For this review, take the finished solid that the model builds, in its own axes (mm). A direction names the side the tool comes from. Give positions to 0.01 mm unless a question says otherwise; leave off trailing zeros. Write each loop counter-clockwise with the first axis right and the second up, starting at its lowest first coordinate (ties: lowest second). Pieces come first, ordered by that corner, then holes. Notation, with made-up numbers: M 24.5,79.25 L 70.5,79.25 A15 ccw 70.5,93.25 Z; hole C 57.5,56.5 d11. An arc over 180 degrees is marked long. Write item = value, one per line.
```python
from build123d import *

# Parameters (mm, degrees)
BOSS_EXTRUDE1_DEPTH = 10


with BuildPart() as part:
    # Sketch1 → Boss-Extrude1 (new, symmetric)
    with BuildSketch(Plane(origin=(0, 0, 0), x_dir=(1, 0, 0), z_dir=(0, 1, 0))):
        with BuildLine():
            Line((1.29375, 0), (1.29375, -4.5))
            Line((1.29375, -4.5), (0.5, -4.5))
            Line((0.5, -4.5), (0.5, 0))
            ThreePointArc((0.5, 0), (0.353553391, 0.353553391), (0, 0.5))
            Line((0, 0.5), (-1.20625, 0.5))
            ThreePointArc((-1.20625, 0.5), (-2.441545823, 1.409259047), (-1.940487786, 2.858965441))
            Line((-1.940487786, 2.858965441), (1.559512214, 5.271465441))
            ThreePointArc((1.559512214, 5.271465441), (2.714013578, 5.429837997), (3.52755254, 4.595506155))
            Line((3.52755254, 4.595506155), (4.524019527, 1.437062839))
            ThreePointArc((4.524019527, 1.437062839), (5.076956782, 1.093325967), (5.500851427, 1.5875))
            Line((5.500851427, 1.5875), (5.500851427, 5.5))
            Line((5.500851427, 5.5), (6.294601427, 5.5))
            Line((6.294601427, 5.5), (6.294601427, 1.5875))
            ThreePointArc((6.294601427, 1.5875), (5.197774033, 0.30882469), (3.767048886, 1.198243845))
            Line((3.767048886, 1.198243845), (2.7705819, 4.356687161))
            ThreePointArc((2.7705819, 4.356687161), (2.456170707, 4.67913425), (2.009986604, 4.617927465))
            Line((2.009986604, 4.617927465), (-1.490013396, 2.205427465))
            ThreePointArc((-1.490013396, 2.205427465), (-1.683659014, 1.645154463), (-1.20625, 1.29375))
            Line((-1.20625, 1.29375), (0, 1.29375))
            ThreePointArc((0, 1.29375), (0.914819398, 0.914819398), (1.29375, 0))
        make_face()
    extrude(amount=BOSS_EXTRUDE1_DEPTH, both=True)


solid = part.part
```
1. For line 1 along X through (y, z) = (-4.75, -3.5); line 2 along X through (y, z) = (4.5, -2.5); line 3 along X through (y, z) = (7, 3.5), list the stretches that pass through material, from the lowest coordinate up. Write a range as from..to.
Responses:
line_1 = -1.01..0.39, 3.04..3.87, 5.5..6.29
line_2 = -2.29..-1.06, 3.36..4.19, 5.5..6.29
line_3 = 0.5..1.29
2. Insertion check: P1, Ø5, axis at y = 0, z = 2, coming from the +X side; P2, Ø2, axis at y = 4.5, z = 1, coming from the -X side; P3, Ø3, axis at y = 6.5, z = 3.5, coming from the +X side. Each pin has a flat end and moves straight along its axis. Give the tip position at first contact, or say it passes through.
Responses:
P1 = 5.7
P2 = 0.5
P3 = 1.29
3. Machinability: for faces 1 (the face through (3.276, 0.14, -2.755)), 2 (the face through (4.02, 0.14, -3.04)), 3 (the face through (0.5, 0, 2)), 4 (the face through (0.284, 0.14, -3.429)), which of the approach directions +Z, -Z, +X, -X, +Y, -Y give a long, thin tool a straight path to every point of the face, cutting with its end or side? Answer none if there is none.
Responses:
face_1 = +Z, +Y, -Y
face_2 = -Z, +Y, -Y
face_3 = +Z, -X, +Y, -Y
face_4 = +Y, -Y
4. The part is to be moulded in two halves that separate along Z. For faces 5 (the face through (0.905, 0.14, -0.925)), 6 (the face through (5.501, 0, -4)), 7 (the face through (2.698, 0.14, -5.435)), say which applies: +Z half, -Z half, draft (parallel to the pull), parting line (faces both ways), or undercut.
Responses:
face_5 = undercut
face_6 = draft
face_7 = -Z half
5. We need section B-B, the plane x = -0.5. Write out the cut boundary in (y, z).
Responses:
outline = M -10,-3.85 L 10,-3.85 L 10,-2.89 L -10,-2.89 Z; M -10,-1.29 L 10,-1.29 L 10,-0.5 L -10,-0.5 Z
6. We need section D-D, the plane z = 3. Write out the cut boundary in (x, y).
Responses:
outline = M 0.5,-10 L 1.29,-10 L 1.29,10 L 0.5,10 Z
7. We need section C-C, the plane z = -3.25. Write out the cut boundary in (x, y).
Responses:
outline = M -1.37,-10 L 0.03,-10 L 0.03,10 L -1.37,10 Z; M 3.12,-10 L 3.95,-10 L 3.95,10 L 3.12,10 Z; M 5.5,-10 L 6.29,-10 L 6.29,10 L 5.5,10 Z
8. We need section A-A, the plane y = -1.5. Write out the cut boundary in (x, z).
Responses:
outline = M -1.94,-2.86 L 1.56,-5.27 A1.29 ccw 3.53,-4.6 L 4.52,-1.44 A0.5 cw 5.5,-1.59 L 5.5,-5.5 L 6.29,-5.5 L 6.29,-1.59 A1.29 ccw 3.77,-1.2 L 2.77,-4.36 A0.5 cw 2.01,-4.62 L -1.49,-2.21 A0.5 cw -1.21,-1.29 L 0,-1.29 A1.29 ccw 1.29,0 L 1.29,4.5 L 0.5,4.5 L 0.5,0 A0.5 cw 0,-0.5 L -1.21,-0.5 A1.29 ccw Z
